Input: part model. Units: mm. Frame: model coordinates. Face numbers are marked on the shaded views. A direction names the side the tool comes from. Give positions to 0.01 mm unless a question says otherwise; leave off trailing zeros. Loops run counter-clockwise (first coordinate to the right, second up) from the corner with the lowest first, then second, coordinate; pieces in that order, holes last. Notation, with made-up numbers: (83.5, 47) -> (134.5, 47) arc R33 cw to (134.5, 77) -> close; hole circle Ø2 at (83, 25.5). An arc over 180 degrees is marked (long way). Answer as a JSON object with one key per item and string values. Group by question number.
```python
from build123d import *

# Parameters (mm, degrees)
SKETCH1_W           = 49.4
SKETCH1_H           = 69.2
SKETCH1_W_2         = 27.4
SKETCH1_H_2         = 47.2
BOSS_EXTRUDE1_DEPTH = 5
SKETCH2_R           = 2
CUT_EXTRUDE1_DEPTH  = 15
BOSS_EXTRUDE2_DEPTH = 49.4
CUT_EXTRUDE2_DEPTH  = 40.952638628
SKETCH5_W           = 27.4
SKETCH5_H           = 47.2
CUT_EXTRUDE3_DEPTH  = 93
CUT_EXTRUDE4_START  = -5
CUT_EXTRUDE4_DEPTH  = 93
SKETCH7_W           = 79.4
SKETCH7_H           = 44.952638628
BOSS_EXTRUDE3_DEPTH = 5
BOSS_EXTRUDE4_DEPTH = 3
CUT_EXTRUDE5_DEPTH  = 1
SKETCH10_R          = 2
CUT_EXTRUDE6_DEPTH  = 5
SKETCH11_W          = 15
SKETCH11_H          = 5
CUT_EXTRUDE7_DEPTH  = 13
CHAMFER1_SIZE       = 2.75
BOSS_EXTRUDE5_DEPTH = 0.5
CHAMFER2_SIZE       = 0.25
FILLET1_R           = 5
CHAMFER3_SIZE       = 1
CHAMFER4_SIZE       = 5


with BuildPart() as part:
    # Sketch1 → Boss-Extrude1 (new body)
    with BuildSketch(Plane.XY):
        Rectangle(SKETCH1_W, SKETCH1_H)
        Rectangle(SKETCH1_W_2, SKETCH1_H_2, mode=Mode.SUBTRACT)
    extrude(amount=-BOSS_EXTRUDE1_DEPTH)

    # Sketch2 → Cut-Extrude1 (cut)
    with BuildSketch(Plane.XY):
        with Locations((19.3, 0)):
            Circle(SKETCH2_R)
        with Locations((-19.3, 0)):
            Circle(SKETCH2_R)
    extrude(amount=-CUT_EXTRUDE1_DEPTH, mode=Mode.SUBTRACT)

    # Sketch4 → Boss-Extrude2 (add)
    with BuildSketch(Plane(origin=(24.7, 0, 0), x_dir=(0, 0, -1), z_dir=(1, 0, 0))):
        Polygon((5, 34.6), (44.952638628, 34.6), (5, -34.6), align=None)
    extrude(amount=-BOSS_EXTRUDE2_DEPTH)

    # Sketch3 → Cut-Extrude2 (cut, through all)
    with BuildSketch(Plane(origin=(0, 0, -5), x_dir=(-1, 0, 0), z_dir=(0, 0, -1))):
        Polygon((-19.3, -4.041451884), (-15.8, -2.020725942), (-15.8, 2.020725942), (-19.3, 4.041451884), (-22.8, 2.020725942), (-22.8, -2.020725942), align=None)
        Polygon((19.3, -4.041451884), (22.8, -2.020725942), (22.8, 2.020725942), (19.3, 4.041451884), (15.8, 2.020725942), (15.8, -2.020725942), align=None)
    extrude(amount=CUT_EXTRUDE2_DEPTH, mode=Mode.SUBTRACT)

    # Sketch5 → Cut-Extrude3 (cut)
    with BuildSketch(Plane.XY.offset(-5)):
        Rectangle(SKETCH5_W, SKETCH5_H)
    extrude(amount=-CUT_EXTRUDE3_DEPTH, mode=Mode.SUBTRACT)

    # Sketch6 → Cut-Extrude4 (cut)
    with BuildSketch(Plane.XY.offset(CUT_EXTRUDE4_START)):
        Polygon((19.7, 29.6), (-19.7, 29.6), (-19.7, 10.045894684), (-10.8, 4.907477288), (-10.8, -4.907477288), (-19.7, -10.045894684), (-19.7, -34.6), (19.7, -34.6), (19.7, -10.045894684), (10.8, -4.907477288), (10.8, 4.907477288), (19.7, 10.045894684), align=None)
    extrude(amount=-CUT_EXTRUDE4_DEPTH, mode=Mode.SUBTRACT)

    # Sketch7 → Boss-Extrude3 (add)
    with BuildSketch(Plane(origin=(0, 34.6, 0), x_dir=(1, 0, 0), z_dir=(0, 1, 0))):
        with Locations((0, 22.476319314)):
            Rectangle(SKETCH7_W, SKETCH7_H)
    extrude(amount=-BOSS_EXTRUDE3_DEPTH)

    # Sketch8 → Boss-Extrude4 (add)
    with BuildSketch(Plane.XZ.offset(-29.6)):
        Polygon((25.7, -25.75277675), (32.2, -29.505553499), (38.7, -25.75277675), (38.7, -18.24722325), (32.2, -14.494446501), (25.7, -18.24722325), align=None)
        Polygon((32.2, -17.958548116), (28.7, -19.979274058), (28.7, -24.020725942), (32.2, -26.041451884), (35.7, -24.020725942), (35.7, -19.979274058), align=None, mode=Mode.SUBTRACT)
        Polygon((-32.2, -14.494446501), (-38.7, -18.24722325), (-38.7, -25.75277675), (-32.2, -29.505553499), (-25.7, -25.75277675), (-25.7, -18.24722325), align=None)
        Polygon((-32.2, -17.958548116), (-35.7, -19.979274058), (-35.7, -24.020725942), (-32.2, -26.041451884), (-28.7, -24.020725942), (-28.7, -19.979274058), align=None, mode=Mode.SUBTRACT)
        Polygon((0, -29.447085128), (-6.5, -33.199861878), (-6.5, -40.705415378), (0, -44.458192127), (6.5, -40.705415378), (6.5, -33.199861878), align=None)
        Polygon((-3.5, -34.931912686), (-3.5, -38.97336457), (0, -40.994090512), (3.5, -38.97336457), (3.5, -34.931912686), (0, -32.911186744), align=None, mode=Mode.SUBTRACT)
    extrude(amount=BOSS_EXTRUDE4_DEPTH)

    # Sketch9 → Cut-Extrude5 (cut)
    with BuildSketch(Plane.XZ.offset(-29.6)):
        Polygon((35.7, -24.020725942), (35.7, -19.979274058), (32.2, -17.958548116), (28.7, -19.979274058), (28.7, -24.020725942), (32.2, -26.041451884), align=None)
        Polygon((3.5, -34.931912686), (0, -32.911186744), (-3.5, -34.931912686), (-3.5, -38.97336457), (0, -40.994090512), (3.5, -38.97336457), align=None)
        Polygon((-28.7, -24.020725942), (-28.7, -19.979274058), (-32.2, -17.958548116), (-35.7, -19.979274058), (-35.7, -24.020725942), (-32.2, -26.041451884), align=None)
    extrude(amount=-CUT_EXTRUDE5_DEPTH, mode=Mode.SUBTRACT)

    # Sketch10 → Cut-Extrude6 (cut, through all)
    with BuildSketch(Plane.XZ.offset(-30.6)):
        with Locations((32.2, -22)):
            Circle(SKETCH10_R)
        with Locations((0, -36.952638628)):
            Circle(SKETCH10_R)
        with Locations((-32.2, -22)):
            Circle(SKETCH10_R)
    extrude(amount=-CUT_EXTRUDE6_DEPTH, mode=Mode.SUBTRACT)

    # Sketch11 → Cut-Extrude7 (cut)
    with BuildSketch(Plane.XY):
        with Locations((32.2, 32.1)):
            Rectangle(SKETCH11_W, SKETCH11_H)
        with Locations((-32.2, 32.1)):
            Rectangle(SKETCH11_W, SKETCH11_H)
    extrude(amount=-CUT_EXTRUDE7_DEPTH, mode=Mode.SUBTRACT)

    # Chamfer1
    chamfer1_edges = [part.edges().sort_by_distance(p)[0] for p in [
        (25.7, 26.6, -22),
        (28.95, 26.6, -27.629165125),
        (35.45, 26.6, -27.629165125),
        (38.7, 26.6, -22),
        (35.45, 26.6, -16.370834875),
        (28.95, 26.6, -16.370834875),
        (-28.95, 26.6, -16.370834875),
        (-35.45, 26.6, -16.370834875),
        (-38.7, 26.6, -22),
        (-35.45, 26.6, -27.629165125),
        (-28.95, 26.6, -27.629165125),
        (-25.7, 26.6, -22),
        (3.25, 26.6, -31.323473503),
        (-3.25, 26.6, -31.323473503),
        (-6.5, 26.6, -36.952638628),
        (-3.25, 26.6, -42.581803753),
        (3.25, 26.6, -42.581803753),
        (6.5, 26.6, -36.952638628),
    ]]
    chamfer(chamfer1_edges, length=CHAMFER1_SIZE)

    # Sketch12 → Boss-Extrude5 (add)
    with BuildSketch(Plane.XZ.offset(-26.6)):
        Polygon((32.2, -26.041451884), (35.7, -24.020725942), (35.7, -19.979274058), (32.2, -17.958548116), (28.7, -19.979274058), (28.7, -24.020725942), align=None)
        Polygon((35.45, -20.123611625), (32.2, -18.24722325), (28.95, -20.123611625), (28.95, -23.876388375), (32.2, -25.75277675), (35.45, -23.876388375), align=None, mode=Mode.SUBTRACT)
        Polygon((3.5, -38.97336457), (3.5, -34.931912686), (0, -32.911186744), (-3.5, -34.931912686), (-3.5, -38.97336457), (0, -40.994090512), align=None)
        Polygon((-3.25, -38.829027003), (0, -40.705415378), (3.25, -38.829027003), (3.25, -35.076250253), (0, -33.199861878), (-3.25, -35.076250253), align=None, mode=Mode.SUBTRACT)
        Polygon((-32.2, -26.041451884), (-28.7, -24.020725942), (-28.7, -19.979274058), (-32.2, -17.958548116), (-35.7, -19.979274058), (-35.7, -24.020725942), align=None)
        Polygon((-35.45, -23.876388375), (-32.2, -25.75277675), (-28.95, -23.876388375), (-28.95, -20.123611625), (-32.2, -18.24722325), (-35.45, -20.123611625), align=None, mode=Mode.SUBTRACT)
    extrude(amount=-BOSS_EXTRUDE5_DEPTH)

    # Chamfer2
    chamfer2_edges = [part.edges().sort_by_distance(p)[0] for p in [
        (35.45, 26.6, -22),
        (33.825, 26.6, -24.814582562),
        (30.575, 26.6, -24.814582562),
        (28.95, 26.6, -22),
        (30.575, 26.6, -19.185417438),
        (33.825, 26.6, -19.185417438),
        (-3.25, 26.6, -36.952638628),
        (-1.625, 26.6, -34.138056066),
        (1.625, 26.6, -34.138056066),
        (3.25, 26.6, -36.952638628),
        (1.625, 26.6, -39.76722119),
        (-1.625, 26.6, -39.76722119),
        (-35.45, 26.6, -22),
        (-33.825, 26.6, -19.185417438),
        (-30.575, 26.6, -19.185417438),
        (-28.95, 26.6, -22),
        (-30.575, 26.6, -24.814582562),
        (-33.825, 26.6, -24.814582562),
    ]]
    chamfer(chamfer2_edges, length=CHAMFER2_SIZE)

    # Fillet1
    fillet1_edges = [part.edges().sort_by_distance(p)[0] for p in [
        (24.7, -34.6, -2.5),
        (-24.7, -34.6, -2.5),
        (-24.7, 34.6, -6.5),
        (24.7, 34.6, -6.5),
    ]]
    fillet(fillet1_edges, radius=FILLET1_R)

    # Chamfer3
    chamfer3_edges = [part.edges().sort_by_distance(p)[0] for p in [
        (0, -34.6, 0),
        (0, 34.6, 0),
        (-24.7, 0, 0),
        (24.7, 0, 0),
        (23.235533906, 33.135533906, 0),
        (-23.235533906, 33.135533906, 0),
        (-23.235533906, -33.135533906, 0),
        (23.235533906, -33.135533906, 0),
    ]]
    chamfer(chamfer3_edges, length=CHAMFER3_SIZE)

    # Chamfer4
    chamfer4_edges = [part.edges().sort_by_distance(p)[0] for p in [
        (-39.7, 32.1, -44.952638628),
        (39.7, 32.1, -44.952638628),
        (39.7, 32.1, -13),
        (-39.7, 32.1, -13),
    ]]
    chamfer(chamfer4_edges, length=CHAMFER4_SIZE)


solid = part.part
```
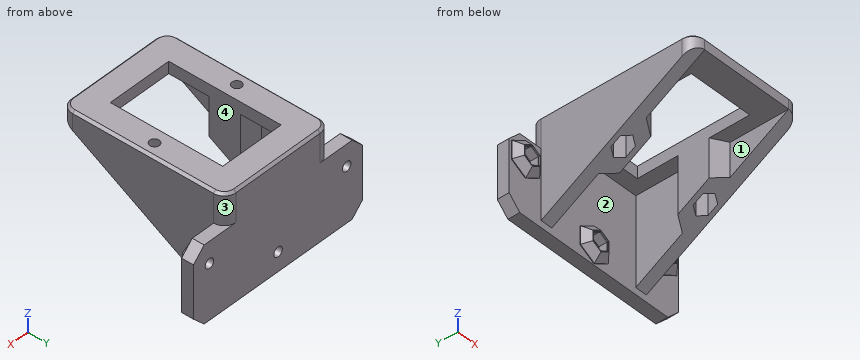
Q1. Section B-B on y = -20. Return the cut outline in (x, z), then the cut area to 3 significant figures.
Q2. Set-up query: the marked faces 1, 2, 3 and 4. Return all of +Z, -Z, +X, -X, +Y, -Y with unobstructed straight access to the full face (end or side cutting, diameter ignored); none if empty.
Q3. Section A-A on x = 7.5. Return the cut outline in (y, z), then the cut area to 3 significant figures.
Q4. Ray query, probe 1 along Z at (x, y) = (0, 33); probe 2 along Y at (x, z) = (-19, -2); probe 3 along X at (y, z) = (15.5, -8). Return the intervals inside material, ascending.
Q5. Section D-D on x = -5. Return the cut outline in (y, z), then the cut area to 3 significant figures.
Q6. Section C-C on y = -27.5. Return the cut outline in (x, z), then the cut area to 3 significant figures.
Q7. Pin query (flat end, axial travel): pin 1 Ø10 at (y, z) = (12.5, -22.5) entering from -X; pin 2 Ø20.5 at (y, z) = (7, -29.5) entering from +X; pin 3 Ø5.5 at (x, y) = (-20, 1.5) entering from -Z. Return the tip coordinate at first contact, or that it passes through.
Numbers:
{
 "1": {"outline": "(-24.7, -13.43) -> (-19.7, -13.43) -> (-19.7, -5) -> (-13.7, -5) -> (-13.7, 0) -> (-23.7, 0) -> (-24.7, -1) -> close; (13.7, -5) -> (19.7, -5) -> (19.7, -13.43) -> (24.7, -13.43) -> (24.7, -1) -> (23.7, 0) -> (13.7, 0) -> close", "area": "193 mm²"},
 "2": {"face 1": "-Z, -Y", "face 2": "none", "face 3": "+Z, +X, +Y", "face 4": "+Z, -Z"},
 "3": {"outline": "(-34.6, -5) -> (-23.6, -5) -> (-23.6, 0) -> (-33.6, 0) -> (-34.6, -1) -> close; (23.6, -5) -> (29.6, -5) -> (29.6, -44.95) -> (34.6, -44.95) -> (34.6, -1) -> (33.6, 0) -> (23.6, 0) -> close", "area": "309 mm²"},
 "4": {"probe 1": "z = -44.95 to -38.95, -34.95 to 0", "probe 2": "y = -34.6 to -1.98, 1.98 to 34.6", "probe 3": "x = -24.7 to -19.7, 19.7 to 24.7"},
 "5": {"outline": "(-34.6, -5) -> (-23.6, -5) -> (-23.6, 0) -> (-33.6, 0) -> (-34.6, -1) -> close; (23.6, -5) -> (29.6, -5) -> (29.6, -32.33) -> (29.35, -32.33) -> (27.85, -34.07) -> (27.85, -39.84) -> (29.35, -41.57) -> (29.6, -41.57) -> (29.6, -44.95) -> (34.6, -44.95) -> (34.6, -1) -> (33.6, 0) -> (23.6, 0) -> close", "area": "322 mm²"},
 "6": {"outline": "(-24.7, -9.1) -> (-19.7, -9.1) -> (-19.7, -5) -> (19.7, -5) -> (19.7, -9.1) -> (24.7, -9.1) -> (24.7, -1) -> (23.7, 0) -> (-23.7, 0) -> (-24.7, -1) -> close", "area": "287 mm²"},
 "7": {"pin 1": "stops at x = -24.7", "pin 2": "stops at x = 24.7", "pin 3": "stops at z = -27.43"}
}
